Autodesk Inventor part; units mm, degrees
ref_plane "YZ Plane" through (0, 0, 0) normal (1, 0, 0) x (0, 1, 0)
ref_plane "XZ Plane" through (0, 0, 0) normal (0, 1, 0) x (-1, 0, 0)
ref_plane "XY Plane" through (0, 0, 0) normal (0, 0, 1) x (1, 0, 0)
sketch "Sketch1" plane through (0, 0, 0) normal (0, 0, 1) x (1, 0, 0)
  circle A0 centre (0, 0) radius 5.715
  dimension "d0" = 11.43
extrude "Extrusion1" add sketch "Sketch1" along normal blind 0.508
sketch "Sketch2" plane through (0, 0, 0.508) normal (0, 0, 1) x (1, 0, 0)
  circle A0 centre (0, 0) radius 5.715
  circle A1 centre (0, 0) radius 5.08
  dimension "d3" = 10.16
extrude "Extrusion2" add sketch "Sketch2" along normal blind 1.27 contours A1
fillet "Fillet1" radius 3.175 1 edges at (-5.08, 0, 1.778)
sketch "Sketch3" plane through (0, 0, 1.778) normal (0, 0, 1) x (1, 0, 0)
  circle A0 centre (0, 0) radius 2.54
  line L0 (2.9329, 0) -> (1.4665, -2.54)
  line L1 (1.4665, -2.54) -> (-1.4665, -2.54)
  line L2 (-1.4665, -2.54) -> (-2.9329, 0)
  line L3 (-2.9329, 0) -> (-1.4665, 2.54)
  line L4 (-1.4665, 2.54) -> (1.4665, 2.54)
  line L5 (1.4665, 2.54) -> (2.9329, 0)
  dimension "d7" = 2.54
extrude "Extrusion3" cut sketch "Sketch3" against normal blind 1.016
sketch "Sketch4" plane through (0, 0, 0) normal (0, 0, -1) x (-1, 0, 0)
  circle A0 centre (0, 0) radius 5.715
  circle A1 centre (0, 0) radius 3.175
  dimension "d10" = 6.35
extrude "Extrusion4" add sketch "Sketch4" along normal blind 12.7 contours A1
thread "Thread1"
properties part number "8020_10series_0.5in_0.25-20_capscrews"
Could you check a few things on this model? Use its own coordinates, in mm. A direction names the side the tool comes from. Coordinates: 2 decimals unless noted, no trailing zeros. Order: outer loops, then holes, each group sorted by start corner. A loop starts at its lowest first (then second) coordinate and runs counter-clockwise, first axis right, second up. Notation, with made-up numbers: M -16,50 L -11,50 A18 ccw -11,73 Z; hole C 46,41 d4. An arc over 180 degrees is marked long. Use one line per item in the form item = value. Start each with the question number.
1. We'd pull the mould along X, two halves only. Please class faces 3 (the cylindrical face through (5.45, -1.72, 0.25)), 4 (the flat face through (2.19, 1.29, 1.28)), 5 (the flat face through (0, 0, -12.7)): +X half, -X half, draft (parallel to the pull), parting line (faces both ways), or undercut.
2. Suppose I cut it at A-A on z = -8.75. Write out the boundary of the cut face in (x, y) (3 decimals), then the cut area to 3 significant figures.
3. For pin 1 (2 mm diameter, centred on y = -2.5, z = -5.5, fed in from -X); pin 2 (1.5 mm diameter, centred on x = -3, z = -9, fed in from -Y); pin 3 (0.8 mm diameter, centred on x = 0.5, z = 1.5, fed in from +Y) (3 decimals), each with a flat end and sliding along its axis, tell me the tip position at first contact or that it passes through.
4. Please list where these lines run through material, in increasing order: line 1 (Z direction, x = 4, y = -3.5); line 2 (Z direction, x = -1.5, y = -0.5); line 3 (Y direction, x = 0.75, z = -8.75).
5. On a 3-axis mill with a long thin cutter (end or side, diameter ignored), from which of +Z, -Z, +X, -X, +Y, -Y can I reach the whole of each face in a straight line? I mean faces 1 (the flat face through (2.5, -2.5, 0)), 2 (the flat face through (2.21, -1.25, 1.28)). Say none if no direction works.
Geometry says:
q1.face_3 = parting line
q1.face_4 = undercut
q1.face_5 = draft
q2.outline = C 0,0 d6.35
q2.area = 31.7 mm^2
q3.pin_1 = -2.8
q3.pin_2 = -2.24
q3.pin_3 = 4.475
q4.line_1 = 0 to 0.51
q4.line_2 = -12.7 to 0.76
q4.line_3 = -3.09 to 3.09
q5.face_1 = -Z
q5.face_2 = +Z
